Part model, mm, in its own coordinate system. Face numbers are marked on the shaded views. A direction names the side the tool comes from. Give positions to 0.01 mm unless a question says otherwise; leave off trailing zeros. Write each loop counter-clockwise with the first axis right and the second up, starting at its lowest first coordinate (ties: lowest second). Pieces come first, ordered by that corner, then holes. Notation, with made-up numbers: M -30.75,25.25 L -7.75,25.25 A30 ccw -7.75,64.25 Z; hole C -2.75,26.5 d1. An arc over 180 degrees is marked long. Use CSV: the item, a comma, the result in double quotes. Start each with the question number.
Item 1: Pin check, flat tips, straight feed: pin 1 (1.7 mm diameter, centred on y = 17.5, z = -30.5, fed in from -X); pin 2 (2 mm diameter, centred on y = 11, z = -2, fed in from +X); pin 3 (6 mm diameter, centred on x = 33, y = 41, fed in from +Z); pin 4 (2 mm diameter, centred on x = 30.26, y = 37.75, fed in from +Z). Stop position of each tip, or through.
Item 2: Which spindle directions (+Z, -Z, +X, -X, +Y, -Y) get a long thin tool onto all of the face, cutting with end or side? Do the marked faces 1 and 2. Say none if no direction does.
Item 3: Cut at B-B (y = 21). List the corners of the cut face in (x, z), then the cut area to 3 significant figures.
Item 4: Drill centre lines: line 1 (X direction, y = 17, z = -13); line 2 (X direction, y = 24, z = -12); line 3 (Z direction, x = 1, y = 13). Where is each one in solid material? Low to high. Write a range as [from, to].
Item 5: Cut at C-C (z = -54.5). List the corners of the cut face in (x, y), then the cut area to 3 significant figures.
Item 6: Cut at A-A (x = 20). List the corners of the cut face in (y, z).
Item 7: Cut at D-D (z = -5). List the corners of the cut face in (x, y).
Item 8: Mould opens along X. For the marked faces 3, 4 and 5 say: released by +X, released by -X, zero draft, split by the parting line, or undercut.
from build123d import *

# Parameters (mm, degrees)
SKETCH3_W           = 40
SKETCH3_H           = 53.7
BOSS_EXTRUDE1_DEPTH = 27.5
BOSS_EXTRUDE4_DEPTH = 27.5
CUT_EXTRUDE1_DEPTH  = 28.5
SKETCH7_R           = 20
CUT_EXTRUDE2_DEPTH  = 54.7
BOSS_EXTRUDE5_DEPTH = 4.5
SKETCH9_R           = 10.5
CUT_EXTRUDE3_DEPTH  = 59.2000001
SKETCH10_R          = 1.85
CUT_EXTRUDE4_DEPTH  = 59.2000001
CUT_EXTRUDE5_DEPTH  = 59.2
CUT_EXTRUDE7_DEPTH  = 59.2000001


with BuildPart() as part:
    # Sketch3 → Boss-Extrude1 (new body)
    with BuildSketch(Plane(origin=(0, 0, 0), x_dir=(1, 0, 0), z_dir=(0, 1, 0))):
        with Locations((20, 26.85)):
            Rectangle(SKETCH3_W, SKETCH3_H)
    extrude(amount=BOSS_EXTRUDE1_DEPTH)

    # Sketch4 → Boss-Extrude4 (add)
    with BuildSketch(Plane(origin=(0, 27.5, 0), x_dir=(1, 0, 0), z_dir=(0, 1, 0))):
        with BuildLine():
            Line((0, 41.2), (0, 33.7))
            ThreePointArc((0, 33.7), (-2.999999474, 37.45), (0, 41.2))
        make_face()
        with BuildLine():
            Line((0, 11.5), (0, 4))
            ThreePointArc((0, 4), (-2.999999474, 7.75), (0, 11.5))
        make_face()
        with BuildLine():
            Line((40, 41.2), (40, 33.7))
            ThreePointArc((40, 33.7), (42.999999474, 37.45), (40, 41.2))
        make_face()
        with BuildLine():
            Line((40, 11.5), (40, 4))
            ThreePointArc((40, 4), (42.999999474, 7.75), (40, 11.5))
        make_face()
    extrude(amount=-BOSS_EXTRUDE4_DEPTH)

    # Sketch6 → Cut-Extrude1 (cut, through all)
    with BuildSketch(Plane(origin=(0, 27.5, 0), x_dir=(1, 0, 0), z_dir=(0, 1, 0))):
        with BuildLine():
            Line((0, 28.15), (0, 16.05))
            ThreePointArc((0, 16.05), (3.100001365, 22.1), (0, 28.15))
        make_face()
        with BuildLine():
            Line((40, 28.15), (40, 16.05))
            ThreePointArc((40, 16.05), (36.899998635, 22.1), (40, 28.15))
        make_face()
    extrude(amount=-CUT_EXTRUDE1_DEPTH, mode=Mode.SUBTRACT)

    # Sketch7 → Cut-Extrude2 (cut, through all)
    with BuildSketch(Plane(origin=(0, 0, -53.7), x_dir=(-1, 0, 0), z_dir=(0, 0, -1))):
        with Locations((-20, 27.5)):
            Circle(SKETCH7_R)
    extrude(amount=-CUT_EXTRUDE2_DEPTH, mode=Mode.SUBTRACT)

    # Sketch8 → Boss-Extrude5 (add)
    with BuildSketch(Plane(origin=(0, 0, -53.7), x_dir=(-1, 0, 0), z_dir=(0, 0, -1))):
        with BuildLine():
            Line((-40, 27.5), (-40, 0))
            Line((-40, 0), (0, 0))
            Line((0, 0), (0, 27.5))
            ThreePointArc((0, 27.5), (-20, 47.5), (-40, 27.5))
        make_face()
    extrude(amount=BOSS_EXTRUDE5_DEPTH)

    # Sketch9 → Cut-Extrude3 (cut, through all)
    with BuildSketch(Plane(origin=(0, 0, -58.2), x_dir=(-1, 0, 0), z_dir=(0, 0, -1))):
        with Locations((-20, 27.5)):
            Circle(SKETCH9_R)
    extrude(amount=-CUT_EXTRUDE3_DEPTH, mode=Mode.SUBTRACT)

    # Sketch10 → Cut-Extrude4 (cut, through all)
    with BuildSketch(Plane(origin=(0, 0, -58.2), x_dir=(-1, 0, 0), z_dir=(0, 0, -1))):
        with Locations((-23.75, 12.9)):
            Circle(SKETCH10_R)
        with Locations((-16.333793604, 14.1)):
            Circle(SKETCH10_R)
        with Locations((-32.995056342, 30.769328778)):
            Circle(SKETCH10_R)
        with Locations((-30.255153544, 37.750942678)):
            Circle(SKETCH10_R)
        with Locations((-9.87, 37.119384527)):
            Circle(SKETCH10_R)
        with Locations((-5.2, 31.25575215)):
            Circle(SKETCH10_R)
    extrude(amount=-CUT_EXTRUDE4_DEPTH, mode=Mode.SUBTRACT)

    # Sketch11 → Cut-Extrude5 (cut, through all)
    with BuildSketch(Plane.XY):
        with BuildLine():
            Line((40, 5), (45.647961317, 5))
            Line((45.647961317, 5), (45.647961317, -3.041494826))
            Line((45.647961317, -3.041494826), (35, -3.041494826))
            Line((35, -3.041494826), (35, 0))
            ThreePointArc((35, 0), (38.535533906, 1.464466094), (40, 5))
        make_face()
    extrude(amount=-CUT_EXTRUDE5_DEPTH, mode=Mode.SUBTRACT)

    # Sketch12 → Cut-Extrude7 (cut, through all)
    with BuildSketch(Plane.XY):
        with BuildLine():
            Line((0, 5), (-3.969490024, 5))
            Line((-3.969490024, 5), (-3.969490024, -1.478021918))
            Line((-3.969490024, -1.478021918), (5, -1.478021918))
            Line((5, -1.478021918), (5, 0))
            ThreePointArc((5, 0), (1.464466094, 1.464466094), (0, 5))
        make_face()
    extrude(amount=-CUT_EXTRUDE7_DEPTH, mode=Mode.SUBTRACT)


solid = part.part
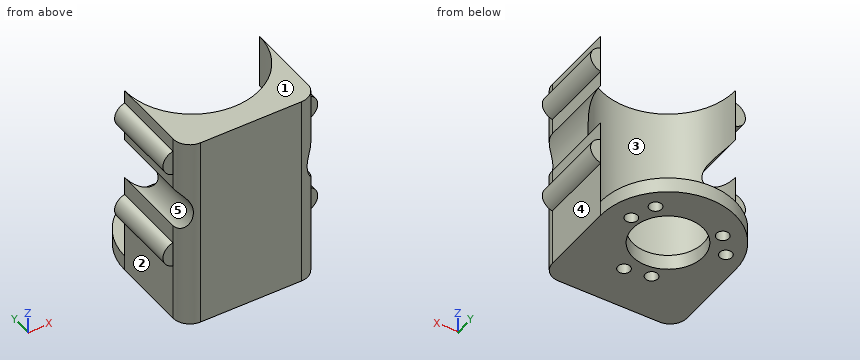
Worked answers:
1,pin 1,"stops at x = 0"
1,pin 2,"stops at x = 40"
1,pin 3,"stops at z = -53.7"
1,pin 4,"passes through"
2,face 1,"+Z, +X, -X, +Y, -Y"
2,face 2,"-Z, -X, +Y, -Y"
3,outline,"M 0,-58.2 L 11.75,-58.2 L 11.75,-53.7 L 1.09,-53.7 L 1.09,-27.2 A7.45 cw 0,-28.15 L 0,-33.7 A3.84 ccw 0,-41.2 Z; M 0,-16.05 A7.45 cw 1.09,-17 L 1.09,0 L 0,0 L 0,-4 A3.84 ccw 0,-11.5 Z; M 28.25,-58.2 L 40,-58.2 L 40,-41.2 A3.84 ccw 40,-33.7 L 40,-28.15 A7.45 cw 38.91,-27.2 L 38.91,-53.7 L 28.25,-53.7 Z; M 38.91,-17 A7.45 cw 40,-16.05 L 40,-11.5 A3.84 ccw 40,-4 L 40,0 L 38.91,0 Z"
3,area,"265 mm^2"
4,line 1,"x = [0, 2.98], [37.02, 40]"
4,line 2,"x = [0, 0.31], [39.69, 40]"
4,line 3,"z = [-58.2, -27.29], [-16.91, 0]"
5,outline,"M 0,5 A5 ccw 5,0 L 35,0 A5 ccw 40,5 L 40,27.5 A20 ccw 0,27.5 Z; hole C 5.2,31.26 d3.7; hole C 9.87,37.12 d3.7; hole C 20,27.5 d21; hole C 16.33,14.1 d3.7; hole C 23.75,12.9 d3.7; hole C 30.26,37.75 d3.7; hole C 33,30.77 d3.7"
5,area,"1,310 mm^2"
6,outline,"M 0,-58.2 L 17,-58.2 L 17,-53.7 L 7.5,-53.7 L 7.5,0 L 0,0 Z; M 38,-58.2 L 47.5,-58.2 L 47.5,-53.7 L 38,-53.7 Z"
7,outline,"M -1.84,5 L 0,5 A5 ccw 5,0 L 35,0 A5 ccw 40,5 L 41.84,5 L 41.84,27.5 L 40,27.5 A20 cw 0,27.5 L -1.84,27.5 Z"
8,face 3,"undercut"
8,face 4,"released by +X"
8,face 5,"released by -X"
